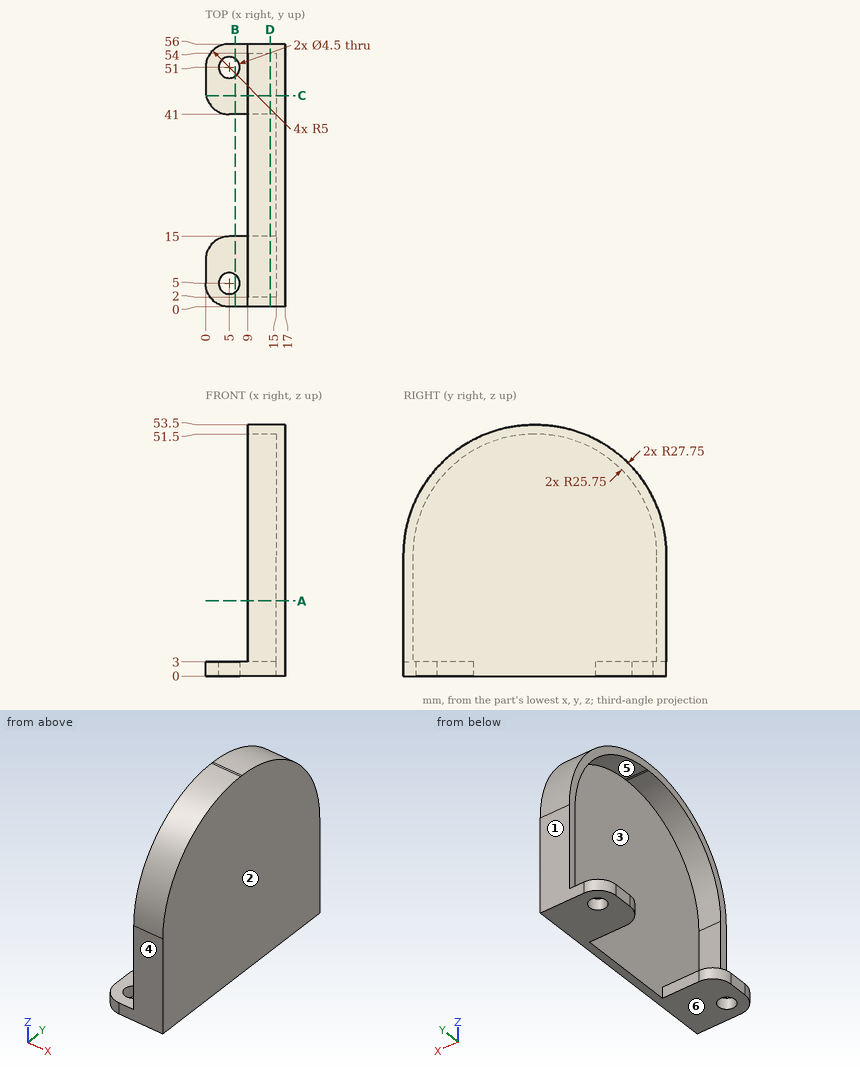
Design review of the part shown in the three views and the two pictorial views. Dimensions are in mm from the part's minimum x, y and z. A direction names the side the tool comes from. Give positions to 0.01 mm unless a question says otherwise; leave off trailing zeros. Loops run counter-clockwise (first coordinate to the right, second up) from the corner with the lowest first, then second, coordinate; pieces in that order, holes last. Notation, with made-up numbers: (64.5, 72.25) - (72.5, 72.25) arc R24 cw to (72.5, 90.25) - close; hole circle Ø1 at (65, 23.25). An arc over 180 degrees is marked (long way). Use CSV: the item, a comma, the result in double quotes. Start each with the question number.
1. Add section C-C (y = 45). State the section outline as (x, z) points.
2. Insertion check: P1, Ø6, axis at x = 11.5, y = 36.5, coming from the -Z side; P2, Ø10, axis at x = 6.5, z = 46.5, coming from the -Y side; P3, Ø1.5, axis at y = 31, z = 43, coming from the -X side; P4, Ø1.5, axis at x = 6.5, z = 11, coming from the -Y side. Each pin has a flat end and moves straight along its axis. Give the tip position at first contact, or say it passes through.
3. Machinability: for the marked faces 5 and 6, which of the approach directions +Z, -Z, +X, -X, +Y, -Y give a long, thin tool a straight path to every point of the face, cutting with its end or side? Answer none if there is none.
4. Add section A-A (z = 16). State the section outline as (x, y) points.
5. Draft analysis for pull direction Y (two halves, no side actions). For the marked faces 1, 2, 3 and 4, state which applies: released by +Y, released by -Y, zero draft, split by the parting line, or undercut.
6. Wall thickness on L1, parallel to Y at x = 5, z = 1.7; L2, parallel to Y at x = 12.5, z = 26.5; L3, parallel to X at y = 18, z = 28: over which ranges is each line inside the solid? List them lowest first.
7. Add section D-D (x = 13.75). State the section outline as (y, z) points, plus the area to 3 significant figures.
8. Add section B-B (x = 6.25). State the section outline as (y, z) points, plus the area to 4 significant figures.
Results found:
1,outline,"(0.1, 0) - (17, 0) - (17, 47.87) - (9, 47.87) - (9, 45.31) - (15, 45.31) - (15, 3) - (0.1, 3) - close"
2,P1,"stops at z = 48.91"
2,P2,"stops at y = 5.38"
2,P3,"stops at x = 15"
2,P4,"passes through"
3,face 5,"-X"
3,face 6,"-Z, +X, -X, +Y, -Y"
4,outline,"(9, 0) - (17, 0) - (17, 56) - (9, 56) - (9, 54) - (15, 54) - (15, 2) - (9, 2) - close"
5,face 1,"released by +Y"
5,face 2,"zero draft"
5,face 3,"undercut"
5,face 4,"released by -Y"
6,L1,"y = 0 to 2.75, 7.25 to 15, 41 to 48.75, 53.25 to 56"
6,L2,"y = 0.01 to 2.01, 53.99 to 55.99"
6,L3,"x = 15 to 17"
7,outline,"(0, 0) - (15, 0) - (15, 3) - (2, 3) - (2, 25.75) arc R25.75 cw to (27.75, 51.5) - (28.25, 51.5) arc R25.75 cw to (54, 25.75) - (54, 3) - (41, 3) - (41, 0) - (56, 0) - (56, 25.75) arc R27.75 ccw to (28.25, 53.5) - (27.75, 53.5) arc R27.75 ccw to (0, 25.75) - close"
7,area,"350 mm²"
8,outline,"(0, 0) - (3.13, 0) - (3.13, 3) - (0, 3) - close; (6.87, 0) - (15, 0) - (15, 3) - (6.87, 3) - close; (41, 0) - (49.13, 0) - (49.13, 3) - (41, 3) - close; (52.87, 0) - (56, 0) - (56, 3) - (52.87, 3) - close"
8,area,"67.55 mm²"
